from build123d import *

# Parameters (mm, degrees)
F1_DEPTH = 63.5
F2_DEPTH = 25.4
F3_DEPTH = 7.9375


with BuildPart() as f1:
    # F0 (on Front) → F1 (new body, symmetric)
    with BuildSketch(Plane.XZ):
        Polygon((22.225, 9.525), (-41.275, 9.525), (-41.275, -9.525), (41.275, -9.525), (41.275, 9.525), align=None)
    extrude(amount=F1_DEPTH, both=True)

    # F0 (on Front) → F2 (join, symmetric)
    with BuildSketch(Plane.XZ):
        with BuildLine():
            Line((22.225, 27.0002), (22.225, 9.525))
            Line((22.225, 9.525), (41.275, 9.525))
            Line((41.275, 9.525), (41.275, 27.0002))
            ThreePointArc((41.275, 27.0002), (45.9246798487, 38.2255201513), (57.15, 42.8752))
            Line((57.15, 42.8752), (60.2788307428, 42.8752))
            Line((60.2788307428, 42.8752), (60.2788307428, 61.9252))
            Line((60.2788307428, 61.9252), (57.15, 61.9252))
            add(Edge.make_bspline(
                [(55.8781690604, 61.9020347807), (56.3029319207, 61.9112789405), (56.7268937511, 61.919000586), (57.15, 61.9252)],
                knots=[110.4402466435, 110.4402466435, 110.4402466435, 110.4402466435, 111.5045361635, 111.5045361635, 111.5045361635, 111.5045361635], degree=3))
            ThreePointArc((55.8781690604, 61.9020347807), (32.0086563549, 51.2420741998), (22.225, 27.0002))
        make_face()
        Polygon((85.7173256435, 61.9252), (60.2788307428, 61.9252), (60.2788307428, 42.8752), (85.6865461387, 42.8752), align=None)
    extrude(amount=F2_DEPTH, both=True)

    # F0 (on Front) → F3 (join, symmetric)
    with BuildSketch(Plane.XZ):
        with BuildLine():
            add(Edge.make_bspline(
                [(-41.275, 9.525), (-40.9017486409, 43.5890820487), (11.8009568178, 60.94277767), (55.8781690604, 61.9020347807)],
                knots=[0, 0, 0, 0, 110.4402466435, 110.4402466435, 110.4402466435, 110.4402466435], degree=3))
            Line((-41.275, 9.525), (22.225, 9.525))
            Line((22.225, 9.525), (22.225, 27.0002))
            ThreePointArc((22.225, 27.0002), (32.0086563549, 51.2420741998), (55.8781690604, 61.9020347807))
        make_face()
    extrude(amount=F3_DEPTH, both=True)

    # F0 (on Front) → F4 (revolve)
    with BuildSketch(Plane.XZ):
        Polygon((85.725, 66.675), (85.7173256435, 61.9252), (85.6865461387, 42.8752), (85.6788307428, 38.1), (111.0788307428, 38.1), (111.0788307428, 66.675), align=None)
    revolve(axis=Axis((85.7019153714, 0, 52.3875), (0.0016157199, 0, 0.9999986947)))


solid = f1.part
The listing builds one solid part. Answer for the finished solid, in the listing's coordinates (mm). A direction names the side the tool comes from. Coordinates: 2 decimals unless noted, no trailing zeros. Loops run counter-clockwise (first coordinate to the right, second up) from the corner with the lowest first, then second, coordinate; pieces in that order, holes last.
1) Find the intervals of material crossed by L1, parallel to Z at x = -18.5, y = 15.5 (3 decimals); L2, parallel to X at y = 23, z = 1 (3 decimals); L3, parallel to Y at x = 28, z = 43, in increasing order.
2) Flat-ended cylindrical pins translate along their axes: pin 1 Ø4 at (x, z) = (43, 58) entering from +Y; pin 2 Ø4 at (y, z) = (8.5, 22) entering from -X; pin 3 Ø16.5 at (x, y) = (-1, 28) entering from +Z (3 decimals). Find the tip coordinate at first contact, or state that the pin passes through.
3) Determine the mould class of faces 6 (the face through (-1, 63.5, 0)), 7 (the face through (45.8, -0.4, 38.1)), 8 (the face through (22.225, 17, 18)) for opening direction X: pulls with the +X half, pulls with the -X half, needs draft (parallel to the pull), parting line crosses it, or undercut.
4) A tool of negligible diameter and unlimited length cuts with its end or side. For faces 1 (the face through (46, -25.4, 42)), 2 (the face through (-3, -7.938, 30)), 3 (the face through (-3, 7.938, 30)), 4 (the face through (46, 25.4, 42)), 5 (the face through (41.275, -1, 4)), from which of +Z, -Z, +X, -X, +Y, -Y can it reach the whole face along a straight path? Write none if from no direction.
5) Find section B-B on y = 39.5. Write down the section's boundary in (x, z) (3 decimals).
6) Find section A-A on z = 3. Write down the section's boundary in (x, y) (3 decimals), then the cut area to 3 significant figures.
Values:
1. L1: z = -9.525 to 9.525
1. L2: x = -41.275 to 41.275
1. L3: y = -25.4 to 25.4
2. pin 1: stops at y = 25.4
2. pin 2: stops at x = -39.36
2. pin 3: stops at z = 9.525
3. face 6: needs draft
3. face 7: undercut
3. face 8: pulls with the -X half
4. face 1: +Z, +X, -X, -Y
4. face 2: +Z, -X, -Y
4. face 3: +Z, -X, +Y
4. face 4: +Z, +X, -X, +Y
4. face 5: -Z, +X, +Y, -Y
5. outline: (-41.275, -9.525) - (41.275, -9.525) - (41.275, 9.525) - (-41.275, 9.525) - close
6. outline: (-41.275, -63.5) - (41.275, -63.5) - (41.275, 63.5) - (-41.275, 63.5) - close
6. area: 10,500 mm2
